Model file for the job. Use its own axes, mm. A direction names the side the tool comes from. Round coordinates to 2 decimals unless told otherwise and drop trailing zeros. Order: outer loops, then holes, each group sorted by start corner. A loop starts at its lowest first (then second) coordinate and runs counter-clockwise, first axis right, second up. Notation, with made-up numbers: (72.25, 13.5) -> (88.25, 13.5) arc R21 cw to (88.25, 34.5) -> close; hole circle Ø1 at (85, 13). An arc over 180 degrees is marked (long way). Use CSV: the item, a comma, the result in double quotes.
```python
from build123d import *

# Parameters (mm, degrees)
SKETCH_1_R          = 2
EXTRUDE_1_DEPTH     = 65
SKETCH_2_R          = 3.515
EXTRUDE_2_DEPTH     = 3
CUT_EXTRUDE_1_DEPTH = 1
CUT_EXTRUDE_1_DRAFT = -12
FILLET_2_R          = 1


with BuildPart() as part:
    # Эскиз1 → Бобышка-Вытянуть1 (new body)
    with BuildSketch(Plane(origin=(0, 0, 0), x_dir=(1, 0, 0), z_dir=(0, 1, 0))):
        with Locations(Location((0, 0, 0), (0, 0, 270))):
            Circle(SKETCH_1_R)
    extrude(amount=EXTRUDE_1_DEPTH)

    # Эскиз2 → Бобышка-Вытянуть2 (add)
    with BuildSketch(Plane(origin=(0, 65, 0), x_dir=(1, 0, 0), z_dir=(0, 1, 0))):
        with Locations(Location((0, 0, 0), (0, 0, 270))):
            Circle(SKETCH_2_R)
    extrude(amount=EXTRUDE_2_DEPTH)


with BuildPart() as cut_extrude_1_tool:
    # Эскиз3 → Вырез-Вытянуть1 (with draft: the straight prism first)
    with BuildSketch(Plane(origin=(0, 68, 0), x_dir=(1, 0, 0), z_dir=(0, 1, 0))):
        Polygon((-2.641549473, 0.422769916), (-2.641549473, -0.422769916), (-0.422769916, -0.422769916), (-0.422769916, -2.641549473), (0.422769916, -2.641549473), (0.422769916, -0.422769916), (2.641549473, -0.422769916), (2.641549473, 0.422769916), (0.422769916, 0.422769916), (0.422769916, 2.641549473), (-0.422769916, 2.641549473), (-0.422769916, 0.422769916), align=None)
    extrude(amount=-CUT_EXTRUDE_1_DEPTH)
    # Вырез-Вытянуть1: the draft: its side faces are tilted about the plane it starts from
    cut_extrude_1_sides = [cut_extrude_1_tool.faces().sort_by_distance(p)[0] for p in [
        (-2.641549473, 67.5, 0),
        (-1.532159694, 67.5, 0.422769916),
        (-0.422769916, 67.5, 1.532159694),
        (0, 67.5, 2.641549473),
        (0.422769916, 67.5, 1.532159694),
        (1.532159694, 67.5, 0.422769916),
        (2.641549473, 67.5, 0),
        (1.532159694, 67.5, -0.422769916),
        (0.422769916, 67.5, -1.532159694),
        (0, 67.5, -2.641549473),
        (-0.422769916, 67.5, -1.532159694),
        (-1.532159694, 67.5, -0.422769916),
    ]]
    draft(cut_extrude_1_sides, Plane(origin=(0, 68, 0), x_dir=(1, 0, 0), z_dir=(0, 1, 0)), CUT_EXTRUDE_1_DRAFT)


with BuildPart() as part_1:
    add(part.part)

    # Вырез-Вытянуть1: cut by cut_extrude_1_tool
    add(cut_extrude_1_tool.part, mode=Mode.SUBTRACT)

    # Скругление2
    # the kernel refuses this fillet: 1 mm, written as the material it takes off along each edge
    with BuildSketch(Plane(origin=(0, 68, 0), x_dir=(0, 0, 1), z_dir=(-1, 0, 0))) as fillet_2_piece_1:
        with BuildLine():
            CenterArc((3.515 - FILLET_2_R, -FILLET_2_R), FILLET_2_R, 0, 90)
            Line((3.515 - FILLET_2_R, 0), (3.515, 0))
            Line((3.515, 0), (3.515, -FILLET_2_R))
        make_face()
    revolve(axis=Axis((0, 68, 0), (0, 1, 0)), mode=Mode.SUBTRACT)


solid = part_1.part
```
Q1. Probe line 1 along Y through (x, z) = (-1.5, 2); line 2 along Z through (x, y) = (-0.5, 14.5); line 3 along Z through (x, y) = (1.25, 60). List the from-to ranges inside material, lowest first.
From the geometry:
line 1,"y = 65 to 68"
line 2,"z = -1.94 to 1.94"
line 3,"z = -1.56 to 1.56"
Q2. Pin check, flat tips, straight feed: pin 1 (1.5 mm diameter, centred on x = -0.5, y = 39, fed in from +Z); pin 2 (1.5 mm diameter, centred on x = -1.5, z = 3, fed in from -Y); pin 3 (2 mm diameter, centred on y = 29, z = -1.5, fed in from +X). Stop position of each tip, or through.
From the geometry:
pin 1,"stops at z = 2"
pin 2,"stops at y = 65"
pin 3,"stops at x = 1.94"
Q3. Which spindle directions (+Z, -Z, +X, -X, +Y, -Y) get a long thin tool onto all of the face, cutting with end or side? Do faces 1 (the flat face through (-1, 68, -1)), 2 (the flat face through (-2, 65, 2)). Say none if no direction does.
From the geometry:
face 1,"+Z, -Z, +X, -X, +Y"
face 2,"-Y"
Q4. Mould opens along X. For faces 3 (the cylindrical face through (-2.14, 65.99, -2.79)), 4 (the flat face through (0, 0, 0)), 5 (the flat face through (0, 67, 0)) say: +X half, -X half, draft (parallel to the pull), parting line (faces both ways), or undercut.
From the geometry:
face 3,"parting line"
face 4,"draft"
face 5,"undercut"
Q5. Cut at A-A (y = 60). Give the cut face in (x, z), plus the area to 3 significant figures.
From the geometry:
outline,"circle Ø4 at (0, 0)"
area,"12.6 mm²"
